Source: three-view drawing plus pictorial views. Frame: mm from the lowest corner of the part. A direction names the side the tool comes from. Give positions to 0.01 mm unless a question says otherwise; leave off trailing zeros. Write each loop counter-clockwise with the first axis right and the second up, starting at its lowest first coordinate (ties: lowest second). Pieces come first, ordered by that corner, then holes. Notation, with made-up numbers: M -23.5,-27.75 L -13.5,-27.75 A25 cw -13.5,-12.75 Z; hole C 30.5,22.5 d5. An arc over 180 degrees is marked long. Return JSON: item names as keys, results as strings.
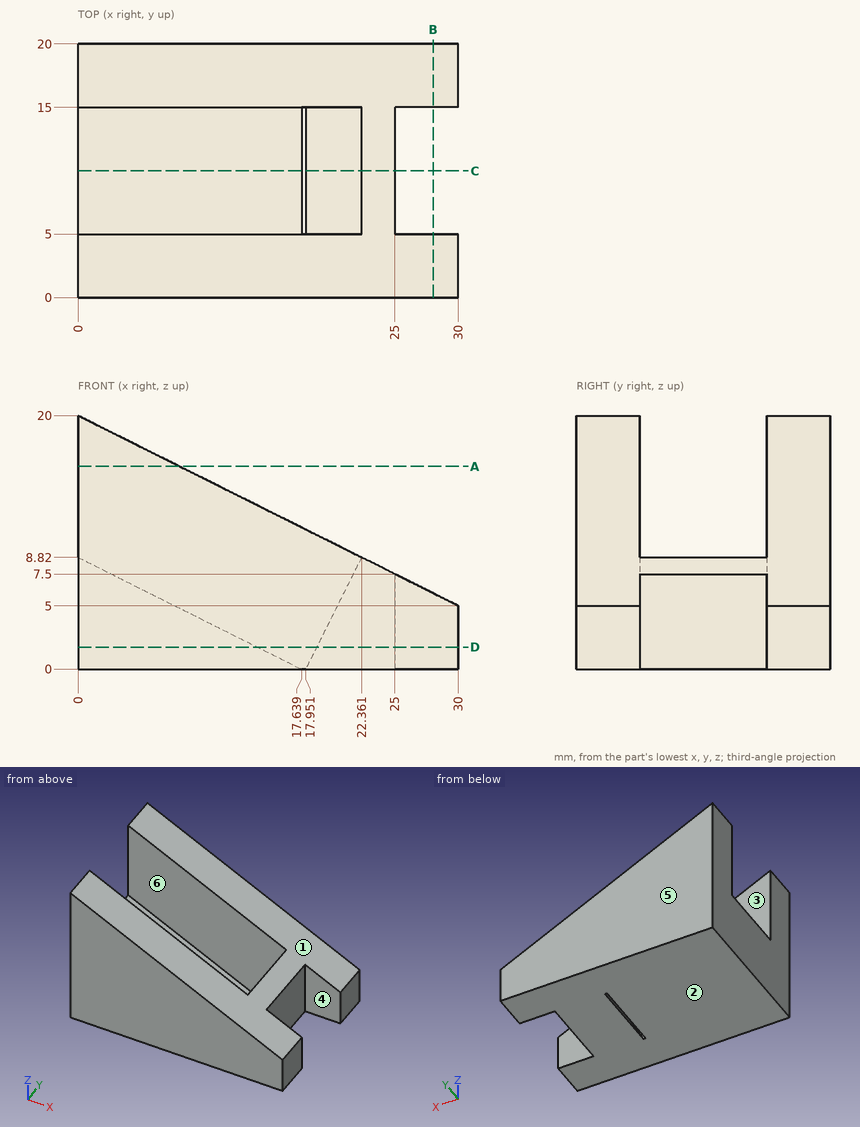
1) Set-up query: the marked faces 4, 5 and 6. Return all of +Z, -Z, +X, -X, +Y, -Y with unobstructed straight access to the full face (end or side cutting, diameter ignored); none if empty.
Numbers:
{"face 4": "+Z, -Z, +X", "face 5": "+Z, -Z, +X, -X, +Y", "face 6": "+Z"}
2) Line query: line 1 (Y direction, x = 14, z = 9.75); line 2 (X direction, y = 7.75, z = 3.5); line 3 (X direction, y = 5.75, z = 2.5). Output: solid intervals per line, ascending. Write a range as [from, to].
Numbers:
{"line 1": "y = [0, 5], [15, 20]", "line 2": "x = [0, 10.64], [19.7, 25]", "line 3": "x = [0, 12.64], [19.2, 25]"}
3) Contact query for flat-ended pins moving along their axis: pin 1 Ø5.5 at (x, z) = (28, 3.5) entering from -Y; pin 2 Ø4 at (y, z) = (12, 3.5) entering from +X; pin 3 Ø1.5 at (y, z) = (7.5, 17.5) entering from -X. Output: stop coordinate, or through.
Numbers:
{"pin 1": "stops at y = 0", "pin 2": "stops at x = 25", "pin 3": "passes through"}
4) Cut plane D-D, the plane z = 1.75. Return the cut outline in (x, y).
Numbers:
{"outline": "M 0,0 L 30,0 L 30,5 L 25,5 L 25,15 L 30,15 L 30,20 L 0,20 Z; hole M 14.14,5 L 18.83,5 L 18.83,15 L 14.14,15 Z"}
5) Draft query along X for the marked faces 1, 2 and 3. Return one class per face: released by +X, released by -X, zero draft, split by the parting line, or undercut.
Numbers:
{"face 1": "released by +X", "face 2": "zero draft", "face 3": "undercut"}
6) Cut plane B-B, the plane x = 28. Return the cut outline in (y, z), then the cut area to 3 significant figures.
Numbers:
{"outline": "M 0,0 L 5,0 L 5,6 L 0,6 Z; M 15,0 L 20,0 L 20,6 L 15,6 Z", "area": "60.0 mm²"}
7) Cut plane C-C, the plane y = 10. Return the cut outline in (x, z).
Numbers:
{"outline": "M 0,0 L 17.64,0 L 0,8.82 Z; M 17.95,0 L 25,0 L 25,7.5 L 22.36,8.82 Z"}
8) Cut plane A-A, the plane z = 16. Return the cut outline in (x, y).
Numbers:
{"outline": "M 0,0 L 8,0 L 8,5 L 0,5 Z; M 0,15 L 8,15 L 8,20 L 0,20 Z"}
